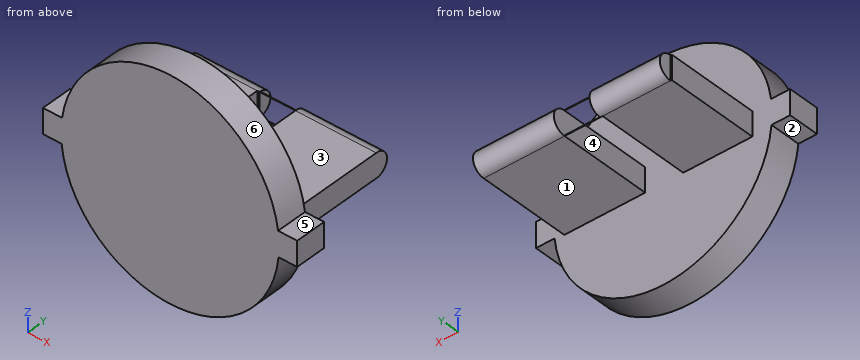
Autodesk Inventor part; units mm, degrees
ref_plane "YZ Plane" through (0, 0, 0) normal (1, 0, 0) x (0, 1, 0)
ref_plane "XZ Plane" through (0, 0, 0) normal (0, 1, 0) x (-1, 0, 0)
ref_plane "XY Plane" through (0, 0, 0) normal (0, 0, 1) x (1, 0, 0)
sketch "Sketch1" plane through (0, 0, 0) normal (0, 1, 0) x (-1, 0, 0)
  line L0 (-34.8245, 0.6257) -> (-40.8245, 0.6257)
  line L1 (-40.8245, 0.6257) -> (-40.8245, 4.6257)
  line L2 (-40.8245, 4.6257) -> (-34.693, 4.6257)
  line L3 (-40.8245, 0.6257) -> (-40.8245, -3.3743)
  line L4 (-40.8245, -3.3743) -> (-34.837, -3.3743)
  line L5 (0, 23.9304) -> (0, -22.2454)
  line L6 (34.8245, 0.6257) -> (40.8245, 0.6257)
  line L7 (40.8245, 0.6257) -> (40.8245, 4.6257)
  line L8 (40.8245, 4.6257) -> (34.693, 4.6257)
  line L9 (40.8245, 0.6257) -> (40.8245, -3.3743)
  line L10 (40.8245, -3.3743) -> (34.837, -3.3743)
  arc A0 (34.693, 4.6257) -> (-34.693, 4.6257) centre (0, 0) ccw
  arc A1 (-34.837, -3.3743) -> (34.837, -3.3743) centre (0, 0) ccw
  point P0 (-34.693, -3.3743)
  point P1 (34.693, -3.3743)
  dimension "d1" = 4
  dimension "d2" = 6
  dimension "d5" = 35
  dimension "d6" = 35
extrude "Extrusion1" add sketch "Sketch1" along normal blind 10
sketch "Sketch2" plane through (0, 10, 0) normal (0, 1, 0) x (1, 0, 0)
  point P0 (0, 0)
sketch "Sketch3" plane through (0, 10, 0) normal (0, 1, 0) x (1, 0, 0)
  point P0 (0, 0)
sketch "Sketch4" plane through (0, 10, 0) normal (0, 1, 0) x (1, 0, 0)
  line L0 (-28.6835, 3.8877) -> (-6.4953, 3.8877)
  line L1 (-6.4953, 3.8877) -> (-6.4953, -3.8877)
  line L2 (-6.4953, -3.8877) -> (-28.6835, -3.8877)
  line L3 (-28.6835, -3.8877) -> (-28.6835, 3.8877)
  line L4 (-28.6835, 3.8877) -> (-6.4953, -3.8877) construction
  line L5 (-6.4953, 3.8877) -> (-28.6835, -3.8877) construction
  line L6 (5.7367, 3.8877) -> (31.7178, 3.8877)
  line L7 (31.7178, 3.8877) -> (31.7178, -3.8877)
  line L8 (31.7178, -3.8877) -> (5.7367, -3.8877)
  line L9 (5.7367, -3.8877) -> (5.7367, 3.8877)
  line L10 (5.7367, 3.8877) -> (31.7178, -3.8877) construction
  line L11 (31.7178, 3.8877) -> (5.7367, -3.8877) construction
  point P0 (0, 0)
  point P1 (-17.5894, 0)
  point P2 (18.7272, 0)
extrude "Extrusion2" add sketch "Sketch4" along normal blind 30
sketch "Sketch5" plane through (31.7178, 10, 3.8877) normal (1, 0, 0) x (0, 0, -1)
  line L0 (7.7754, 30) -> (0, 30)
  arc A0 (7.7754, 30) -> (0, 30) centre (3.8877, 30.1095) ccw
  point P0 (3.8877, -10)
extrude "Extrusion3" add sketch "Sketch5" against normal blind 60
sketch "Sketch6" plane through (0, 10, 0) normal (0, 1, 0) x (1, 0, 0)
  line L0 (5.7367, -3.8877) -> (5.7367, 3.8877)
  line L1 (-5.7367, 3.8877) -> (5.7367, 3.8877)
  line L2 (5.7367, 3.8877) -> (5.7367, -3.8877)
  line L3 (5.7367, -3.8877) -> (-5.7367, -3.8877)
  line L4 (-5.7367, -3.8877) -> (-5.7367, 3.8877)
  line L5 (-5.7367, 3.8877) -> (5.7367, -3.8877) construction
  line L6 (5.7367, 3.8877) -> (-5.7367, -3.8877) construction
  point P0 (0, 0)
extrude "Extrusion4" cut sketch "Sketch6" along normal blind 60
properties part number "joy part 2"
CAD build for the part. Positions are in the model's coordinates, mm. Face numbers are marked on the shaded views. A direction names the side the tool comes from. Round coordinates to 2 decimals unless told otherwise and drop trailing zeros. Order: outer loops, then holes, each group sorted by start corner. A loop starts at its lowest first (then second) coordinate and runs counter-clockwise, first axis right, second up. Notation, with made-up numbers: (-24.5, 84.25) -> (-10.5, 84.25) arc R36 ccw to (-10.5, 119.25) -> close; hole circle Ø4 at (-39, 56). An arc over 180 degrees is marked (long way). Write item = value, one per line.
(1) Drill centre lines: L1, parallel to X at y = 13.5, z = -3; L2, parallel to Z at x = -9, y = 25; L3, parallel to Y at x = -8.5, z = 10.5. Where is each one in solid material? Low to high.
Answers follow:
L1 = -28.68 to -6.5, 5.74 to 31.72
L2 = -3.89 to 3.89
L3 = 0 to 10
(2) Flat gauge pins, fed straight in: P1, Ø1.8, axis at x = -37.5, y = 7, coming from the -Z side; P2, Ø6, axis at y = 18, z = -1.5, coming from the +X side; P3, Ø12, axis at x = 6.5, z = 23, coming from the +Y side; P4, Ø12, axis at x = -19, z = -9, coming from the -Y side. Where does each tip first touch, or does it go through?
Answers follow:
P1 = -3.37
P2 = 31.72
P3 = 10
P4 = 0
(3) 3-axis set-ups, long thin cutter, end or side, ignore diameter. For the marked faces 1, 2 and 3: which of +Z, -Z, +X, -X, +Y, -Y reach the whole face in a straight line?
Answers follow:
face_1 = -Z, +X, -X, +Y
face_2 = -Z, -X, +Y, -Y
face_3 = +Z, +X, -X, +Y
(4) Cut at B-B (y = 26.5). Write the cut outline in (x, z), plus the area to 3 significant figures.
Answers follow:
outline = (-28.68, -3.89) -> (-6.5, -3.89) -> (-6.5, 3.89) -> (-28.68, 3.89) -> close; (5.74, -3.89) -> (31.72, -3.89) -> (31.72, 3.89) -> (5.74, 3.89) -> close
area = 375 mm²
(5) Pull direction X, two halves, no side cores. Call the marked faces 4, 5 and 6: +X half, -X half, draft (parallel to the pull), parting line (faces both ways), or undercut.
Answers follow:
face_4 = undercut
face_5 = draft
face_6 = parting line
(6) Cut at D-D (x = 26). Write the cut outline in (y, z), plus the area to 3 significant figures.
Answers follow:
outline = (0, -23.43) -> (10, -23.43) -> (10, -3.89) -> (40, -3.89) arc R3.89 ccw (long way) to (40, 3.89) -> (10, 3.89) -> (10, 23.43) -> (0, 23.43) -> close
area = 726 mm²
(7) Cut at C-C (z = 0). Write the cut outline in (x, y).
Answers follow:
outline = (-40.82, 0) -> (40.82, 0) -> (40.82, 10) -> (31.72, 10) -> (31.72, 44) -> (5.74, 44) -> (5.74, 10) -> (-6.5, 10) -> (-6.5, 40) -> (-5.74, 40) -> (-5.74, 44) -> (-28.28, 44) -> (-28.28, 40) -> (-28.68, 40) -> (-28.68, 10) -> (-40.82, 10) -> close
